from build123d import *

# Parameters (mm, degrees)
SKETCH_1_W          = 3
SKETCH_1_H          = 32.905807398
EXTRUDE_1_DEPTH     = 1158
SKETCH_2_W          = 3
SKETCH_2_H          = 16.828171787
SKETCH_2_W_2        = 2.99
CUT_EXTRUDE_1_DEPTH = 3


with BuildPart() as part:
    # 草图1 → 凸台-拉伸1 (new body)
    with BuildSketch(Plane.XY):
        with Locations((-45.625456821, 5.194351007)):
            Rectangle(SKETCH_1_W, SKETCH_1_H)
    extrude(amount=EXTRUDE_1_DEPTH)

    # 草图2 → 切除-拉伸1 (cut)
    with BuildSketch(Plane.ZY.offset(47.125456821)):
        with Locations((1.51, -2.844466799)):
            Rectangle(SKETCH_2_W, SKETCH_2_H)
        with Locations((8.51, -2.844466799)):
            Rectangle(SKETCH_2_W, SKETCH_2_H)
        with BuildLine():
            Line((45, -2.352745294), (115, -2.352745294))
            ThreePointArc((115, -2.352745294), (123, 5.647254706), (115, 13.647254706))
            Line((115, 13.647254706), (45, 13.647254706))
            ThreePointArc((45, 13.647254706), (37, 5.647254706), (45, -2.352745294))
        make_face()
        with Locations((133.51, -2.844466799)):
            Rectangle(SKETCH_2_W, SKETCH_2_H)
        with BuildLine():
            Line((171, -2.352745294), (241, -2.352745294))
            ThreePointArc((241, -2.352745294), (249, 5.647254706), (241, 13.647254706))
            Line((241, 13.647254706), (171, 13.647254706))
            ThreePointArc((171, 13.647254706), (163, 5.647254706), (171, -2.352745294))
        make_face()
        with Locations((258.51, -2.844466799)):
            Rectangle(SKETCH_2_W, SKETCH_2_H)
        with BuildLine():
            Line((297, -2.352745294), (367, -2.352745294))
            ThreePointArc((367, -2.352745294), (375, 5.647254706), (367, 13.647254706))
            Line((367, 13.647254706), (297, 13.647254706))
            ThreePointArc((297, 13.647254706), (289, 5.647254706), (297, -2.352745294))
        make_face()
        with Locations((383.51, -2.844466799)):
            Rectangle(SKETCH_2_W, SKETCH_2_H)
        with BuildLine():
            Line((423, -2.352745294), (493, -2.352745294))
            ThreePointArc((493, -2.352745294), (501, 5.647254706), (493, 13.647254706))
            Line((493, 13.647254706), (423, 13.647254706))
            ThreePointArc((423, 13.647254706), (415, 5.647254706), (423, -2.352745294))
        make_face()
        with Locations((508.51, -2.844466799)):
            Rectangle(SKETCH_2_W, SKETCH_2_H)
        with BuildLine():
            Line((549, -2.352745294), (619, -2.352745294))
            ThreePointArc((619, -2.352745294), (627, 5.647254706), (619, 13.647254706))
            Line((619, 13.647254706), (549, 13.647254706))
            ThreePointArc((549, 13.647254706), (541, 5.647254706), (549, -2.352745294))
        make_face()
        with Locations((633.51, -2.844466799)):
            Rectangle(SKETCH_2_W, SKETCH_2_H)
        with BuildLine():
            Line((675, -2.352745294), (745, -2.352745294))
            ThreePointArc((745, -2.352745294), (753, 5.647254706), (745, 13.647254706))
            Line((745, 13.647254706), (675, 13.647254706))
            ThreePointArc((675, 13.647254706), (667, 5.647254706), (675, -2.352745294))
        make_face()
        with Locations((758.51, -2.844466799)):
            Rectangle(SKETCH_2_W, SKETCH_2_H)
        with Locations((761.51, -2.844466799)):
            Rectangle(SKETCH_2_W, SKETCH_2_H)
        with BuildLine():
            Line((801, -2.352745294), (871, -2.352745294))
            ThreePointArc((871, -2.352745294), (879, 5.647254706), (871, 13.647254706))
            Line((871, 13.647254706), (801, 13.647254706))
            ThreePointArc((801, 13.647254706), (793, 5.647254706), (801, -2.352745294))
        make_face()
        with Locations((886.51, -2.844466799)):
            Rectangle(SKETCH_2_W, SKETCH_2_H)
        with BuildLine():
            Line((927, -2.352745294), (997, -2.352745294))
            ThreePointArc((997, -2.352745294), (1005, 5.647254706), (997, 13.647254706))
            Line((997, 13.647254706), (927, 13.647254706))
            ThreePointArc((927, 13.647254706), (919, 5.647254706), (927, -2.352745294))
        make_face()
        with Locations((1011.51, -2.844466799)):
            Rectangle(SKETCH_2_W, SKETCH_2_H)
        with BuildLine():
            Line((1053, -2.352745294), (1123, -2.352745294))
            ThreePointArc((1123, -2.352745294), (1131, 5.647254706), (1123, 13.647254706))
            Line((1123, 13.647254706), (1053, 13.647254706))
            ThreePointArc((1053, 13.647254706), (1045, 5.647254706), (1053, -2.352745294))
        make_face()
        with Locations((1136.51, -2.844466799)):
            Rectangle(SKETCH_2_W, SKETCH_2_H)
        with Locations((1156.505, -2.844466799)):
            Rectangle(SKETCH_2_W_2, SKETCH_2_H)
    extrude(amount=-CUT_EXTRUDE_1_DEPTH, mode=Mode.SUBTRACT)


solid = part.part
Check sheet for the modelled part. Datum: model origin and axes. Units: mm. Coordinates: 2 decimals unless noted, no trailing zeros. Write each loop counter-clockwise with the first axis right and the second up, starting at its lowest first coordinate (ties: lowest second). Pieces come first, ordered by that corner, then holes.
Item 1: Cross-section at B-B on x = -45.45. Count the separate pieces of the cut face and the enclosed holes in it, then the cut area to 3 significant figures.
Numbers:
separate pieces: 1
enclosed holes: 9
area: 25,600 mm2
Item 2: Scan lines: probe 1 along Y at (x, z) = (-46.5, 620); probe 2 along Y at (x, z) = (-44.4, 966). Record each from-to range of solid material in increasing order.
Numbers:
probe 1: y = -11.26 to -2.29, 13.58 to 21.65
probe 2: y = -11.26 to -2.35, 13.65 to 21.65
Item 3: Depth check by flat-ended pin: pin 1 Ø0.9 at (x, y) = (-45, 0) entering from +Z; pin 2 Ø1.5 at (x, z) = (-45.5, 2) entering from -Y. Enter the tip coordinate at first touch or a pass-through.
Numbers:
pin 1: stops at z = 1155.01
pin 2: stops at y = 5.57
Item 4: Cross-section at A-A on z = 963. Record the boundary of the cut face in (x, y).
Numbers:
outline: (-47.13, -11.26) - (-44.13, -11.26) - (-44.13, -2.35) - (-47.13, -2.35) - close; (-47.13, 13.65) - (-44.13, 13.65) - (-44.13, 21.65) - (-47.13, 21.65) - close
